CAD build for the part. Positions are in the model's coordinates, mm. Round coordinates to 2 decimals unless told otherwise and drop trailing zeros. Order: outer loops, then holes, each group sorted by start corner. A loop starts at its lowest first (then second) coordinate and runs counter-clockwise, first axis right, second up. Notation, with made-up numbers: M 1.5,44.5 L 51.5,44.5 A36 cw 51.5,80.5 Z; hole C 77,49.5 d6. An arc over 180 degrees is marked long. Put each result on its own line as item: value.
```python
from build123d import *

# Parameters (mm, degrees)
F0_W     = 177.8
F0_H     = 66.675
F1_DEPTH = 30.1752
F2_R     = 1.5875
F3_DEPTH = 3.175
F5_DEPTH = 19.05
F6_R     = 3.175
F7_DEPTH = 6.35
F8_R     = 2.3876
F9_DEPTH = 6.35


with BuildPart() as f1:
    # F0 (on Top) → F1 (new body)
    with BuildSketch(Plane.XY):
        Rectangle(F0_W, F0_H)
    extrude(amount=F1_DEPTH)

    # F2 (on face) → F3 (cut)
    with BuildSketch(Plane.XY.offset(30.1752)):
        with Locations((-73.025, 7.9375)):
            Circle(F2_R)
        with Locations((-53.975, 7.9375)):
            Circle(F2_R)
        with Locations((-53.975, -30.1625)):
            Circle(F2_R)
        with Locations((-73.025, -30.1625)):
            Circle(F2_R)
    extrude(amount=-F3_DEPTH, mode=Mode.SUBTRACT)

    # F4 (on face) → F5 (cut)
    with BuildSketch(Plane.XY.offset(30.1752)):
        with BuildLine():
            Line((-58.7375, -25.3873), (-58.7375, 3.1623))
            ThreePointArc((-58.7375, 3.1623), (-63.5, 7.9248), (-68.2625, 3.1623))
            Line((-68.2625, 3.1623), (-68.2625, -25.3873))
            ThreePointArc((-68.2625, -25.3873), (-63.5, -30.1498), (-58.7375, -25.3873))
        make_face()
    extrude(amount=-F5_DEPTH, mode=Mode.SUBTRACT)

    # F6 (on face) → F7 (cut)
    with BuildSketch(Plane.XY.offset(30.1752)):
        with Locations((-26.9748, 1.6129)):
            Circle(F6_R)
        with Locations((23.8252, 1.6129)):
            Circle(F6_R)
        with Locations((23.8252, -22.2123)):
            Circle(F6_R)
        with Locations((-26.9748, -22.2123)):
            Circle(F6_R)
    extrude(amount=-F7_DEPTH, mode=Mode.SUBTRACT)

    # F8 (on face) → F9 (cut)
    with BuildSketch(Plane.XZ.offset(33.3375)):
        with Locations((-63.5, 15.0876)):
            Circle(F8_R)
    extrude(amount=-F9_DEPTH, mode=Mode.SUBTRACT)


solid = f1.part
```
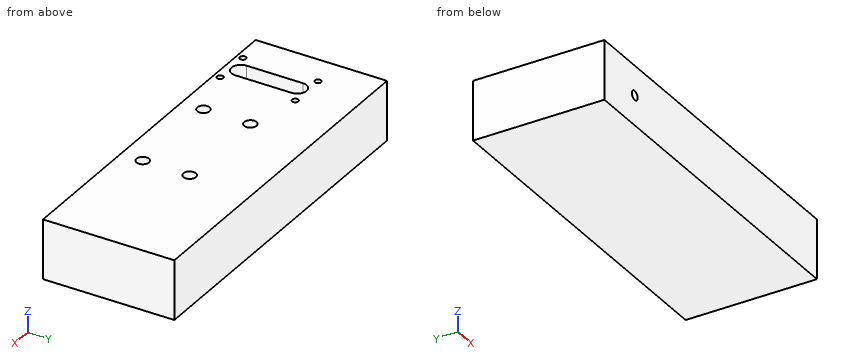
Item 1: Band-saw the part on A-A on x = -63.5. Give the cut face in (y, z).
Answers below:
outline: M -33.34,0 L 33.34,0 L 33.34,30.18 L 7.92,30.18 L 7.92,11.13 L -30.15,11.13 L -30.15,12.7 L -33.34,12.7 Z; M -33.34,17.48 L -30.15,17.48 L -30.15,30.18 L -33.34,30.18 Z
Item 2: Pin check, flat tip, straight feed: P1, Ø3, axis at x = 23, y = 3, coming from the +Z side. Stop position of the tip, or through.
Answers below:
P1: z = 23.83
Item 3: Band-saw the part on B-B on x = -26. Give the cut face in (y, z), and give its area (3 significant figures).
Answers below:
outline: M -33.34,0 L 33.34,0 L 33.34,30.18 L 4.63,30.18 L 4.63,23.83 L -1.41,23.83 L -1.41,30.18 L -19.19,30.18 L -19.19,23.83 L -25.23,23.83 L -25.23,30.18 L -33.34,30.18 Z
area: 1,940 mm²
Item 4: Probe line 1 along X through (y, z) = (0.5, 26); line 2 along Z through (x, y) = (-63.5, -32.05); line 3 along X through (y, z) = (-3, 13). List the from-to ranges inside material, lowest first. Write a range as [from, to].
Answers below:
line 1: [-88.9, -68.26], [-58.74, -29.95], [-24, 20.85], [26.8, 88.9]
line 2: [0, 12.7], [17.48, 30.18]
line 3: [-88.9, -68.26], [-58.74, 88.9]
